Verification items for the finished model (mm, model axes). Face numbers are marked on the shaded views. A direction names the side the tool comes from. Give positions to 0.01 mm unless a question says otherwise; leave off trailing zeros. Write each loop counter-clockwise with the first axis right and the second up, starting at its lowest first coordinate (ties: lowest second). Pieces come first, ordered by that corner, then holes. Notation, with made-up numbers: (-5.5, 29.25) - (10.5, 29.25) arc R4 ccw to (10.5, 36.25) - close; hole circle Ø2 at (23, 31). An arc over 180 degrees is marked (long way). Put each result on its own line as item: value.
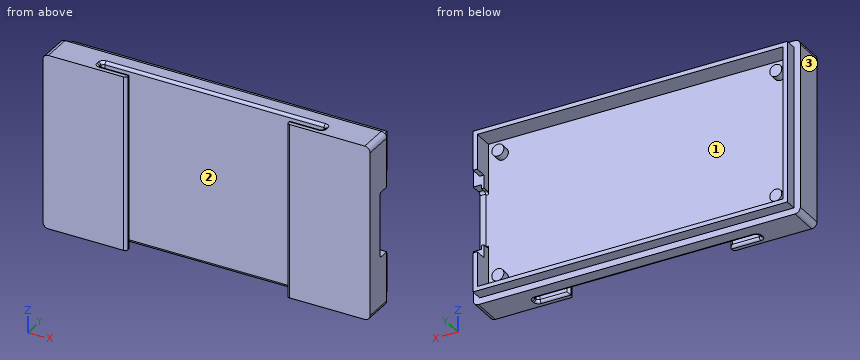
from build123d import *

# Parameters (mm, degrees)
SKETCH2_W               = 61.2
SKETCH2_H               = 32.7
BOSS_EXTRUDE1_DEPTH     = 1.5
BOSS_EXTRUDE2_START     = 1.5
SKETCH2_3_R             = 1.125
BOSS_EXTRUDE2_DEPTH     = 1.5
SKETCH2_4_W             = 61.2
SKETCH2_4_H             = 32.7
BOSS_EXTRUDE3_DEPTH     = 2.5
FILLET1_R               = 1
CUT_EXTRUDE1_DEPTH      = 35.823591142
CUT_EXTRUDE1_DEPTH_BACK = 35.823591142
SKETCH3_W               = 42
SKETCH3_H               = 1.4
SKETCH3_W_2             = 20
SKETCH3_H_2             = 1.25
CUT_EXTRUDE3_DEPTH      = 35.823591142
CUT_EXTRUDE3_DEPTH_BACK = 35.823591142
SKETCH3_4_W             = 5
SKETCH3_4_H             = 1.25
SKETCH3_4_W_2           = 20
FILLET2_R               = 0.5
CUT_EXTRUDE2_START      = 0.75
SKETCH2_5_W             = 1.5
SKETCH2_5_H             = 0.75
SKETCH2_5_H_2           = 10.7
CUT_EXTRUDE2_DEPTH      = 2.25
FILLET3_R               = 0.5
BOSS_EXTRUDE4_DEPTH     = 2.2


with BuildPart() as part:
    # Sketch2 → Boss-Extrude1 (new body)
    with BuildSketch(Plane(origin=(0, 0, 0), x_dir=(1, 0, 0), z_dir=(0, 1, 0))):
        Rectangle(SKETCH2_W, SKETCH2_H)
    extrude(amount=BOSS_EXTRUDE1_DEPTH)

    # Sketch2<3> → Boss-Extrude2 (add)
    with BuildSketch(Plane(origin=(0, 0, 0), x_dir=(1, 0, 0), z_dir=(0, 1, 0)).offset(BOSS_EXTRUDE2_START)):
        Polygon((-30.6, 16.35), (-30.6, -16.35), (30.6, -16.35), (30.6, -6.1), (29.1, -6.1), (29.1, -5.35), (28.6, -5.35), (28.6, -14.35), (-28.6, -14.35), (-28.6, 14.35), (28.6, 14.35), (28.6, 5.35), (30.6, 5.35), (30.6, 16.35), align=None)
        with Locations(Location((-26, 11.75, 0), (0, 0, 270))):
            Circle(SKETCH2_3_R)
        with Locations(Location((-26, -11.75, 0), (0, 0, 270))):
            Circle(SKETCH2_3_R)
        with Locations(Location((26, -11.75, 0), (0, 0, 270))):
            Circle(SKETCH2_3_R)
        with Locations(Location((26, 11.75, 0), (0, 0, 270))):
            Circle(SKETCH2_3_R)
    extrude(amount=BOSS_EXTRUDE2_DEPTH)

    # Sketch2<4> → Boss-Extrude3 (add)
    with BuildSketch(Plane(origin=(0, 0, 0), x_dir=(1, 0, 0), z_dir=(0, 1, 0))):
        Rectangle(SKETCH2_4_W, SKETCH2_4_H)
    extrude(amount=-BOSS_EXTRUDE3_DEPTH)

    # Fillet1
    fillet1_edges = [part.edges().sort_by_distance(p)[0] for p in [
        (-30.6, 0.25, -16.35),
        (30.6, 0.25, -16.35),
        (30.6, 0.25, 16.35),
        (-30.6, 0.25, 16.35),
    ]]
    fillet(fillet1_edges, radius=FILLET1_R)

    # Sketch3 → Cut-Extrude1 (cut, two sides: drawn at the far end of the back side and taken through both)
    with BuildSketch(Plane.XY.offset(-CUT_EXTRUDE1_DEPTH_BACK)):
        with Locations((0, -0.55)):
            Rectangle(SKETCH3_W, SKETCH3_H)
        with Locations((0, -1.875)):
            Rectangle(SKETCH3_W_2, SKETCH3_H_2)
    extrude(amount=CUT_EXTRUDE1_DEPTH + CUT_EXTRUDE1_DEPTH_BACK, mode=Mode.SUBTRACT)

    # Sketch3<4> → Cut-Extrude3 (cut, two sides: drawn at the far end of the back side and taken through both)
    with BuildSketch(Plane.XY.offset(-CUT_EXTRUDE3_DEPTH_BACK)):
        with Locations((12.5, -1.875)):
            Rectangle(SKETCH3_4_W, SKETCH3_4_H)
        with Locations((0, -1.875)):
            Rectangle(SKETCH3_4_W_2, SKETCH3_4_H)
        with Locations((-12.5, -1.875)):
            Rectangle(SKETCH3_4_W, SKETCH3_4_H)
    extrude(amount=CUT_EXTRUDE3_DEPTH + CUT_EXTRUDE3_DEPTH_BACK, mode=Mode.SUBTRACT)

    # Fillet2
    fillet2_edges = [part.edges().sort_by_distance(p)[0] for p in [
        (-18, -1.25, -16.35),
        (-21, -1.25, 0),
        (-21, -0.55, 16.35),
        (-21, 0.15, 0),
        (0, 0.15, 16.35),
        (21, 0.15, 0),
        (21, -0.55, -16.35),
        (21, -1.25, 0),
        (-21, -0.55, -16.35),
        (0, 0.15, -16.35),
        (-18, -1.25, 16.35),
        (21, -0.55, 16.35),
        (18, -1.25, -16.35),
        (18, -1.25, 16.35),
        (-15, -1.25, 0),
        (15, -2.5, 0),
        (-15, -2.5, 0),
        (15, -1.25, 0),
    ]]
    fillet(fillet2_edges, radius=FILLET2_R)

    # Sketch2<5> → Cut-Extrude2 (cut)
    with BuildSketch(Plane(origin=(0, 0, 0), x_dir=(1, 0, 0), z_dir=(0, 1, 0)).offset(CUT_EXTRUDE2_START)):
        with Locations((29.85, 5.725)):
            Rectangle(SKETCH2_5_W, SKETCH2_5_H)
        with Locations((29.85, 0)):
            Rectangle(SKETCH2_5_W, SKETCH2_5_H_2)
        with Locations((29.85, -5.725)):
            Rectangle(SKETCH2_5_W, SKETCH2_5_H)
    extrude(amount=CUT_EXTRUDE2_DEPTH, mode=Mode.SUBTRACT)

    # Fillet3
    fillet3_edges = [part.edges().sort_by_distance(p)[0] for p in [
        (29.85, 0.75, 6.1),
        (29.85, 0.75, -6.1),
        (28.85, 1.5, -5.35),
        (28.85, 1.5, 5.35),
    ]]
    fillet(fillet3_edges, radius=FILLET3_R)

    # Sketch4 → Boss-Extrude4 (add)
    with BuildSketch(Plane(origin=(0, 3, 0), x_dir=(1, 0, 0), z_dir=(0, 1, 0))):
        Polygon((29.4, 15.15), (-29.4, 15.15), (-29.4, -15.15), (29.4, -15.15), (29.4, -7.8), (28.6, -7.8), (28.6, -14.35), (-28.6, -14.35), (-28.6, 14.35), (28.6, 14.35), (28.6, 7.8), (29.4, 7.8), align=None)
    extrude(amount=BOSS_EXTRUDE4_DEPTH)


solid = part.part
Q1. Set-up check for the marked faces 1, 2 and 3: record each of +Z, -Z, +X, -X, +Y, -Y from which the full face is reachable in a straight line by a thin tool's end or side.
Answers follow:
face 1: +Y
face 2: +Z, -Z
face 3: +Z, -Z, -X, +Y, -Y
Q2. Section check A-A, the plane x = -18. Record the cut outline in (y, z), plus the area to 3 significant figures.
Answers follow:
outline: (-2.5, -16.35) - (-1.75, -16.35) arc R0.5 ccw to (-1.25, -15.85) - (-1.25, 15.85) arc R0.5 ccw to (-1.75, 16.35) - (-2.5, 16.35) - close; (0.15, -15.85) arc R0.5 ccw to (0.65, -16.35) - (3, -16.35) - (3, -15.15) - (5.2, -15.15) - (5.2, -14.35) - (1.5, -14.35) - (1.5, 14.35) - (5.2, 14.35) - (5.2, 15.15) - (3, 15.15) - (3, 16.35) - (0.65, 16.35) arc R0.5 ccw to (0.15, 15.85) - close
area: 94.3 mm2
Q3. Section check C-C, the plane x = -3. Record the cut outline in (y, z), plus the area to 3 significant figures.
Answers follow:
outline: (0.15, -15.85) arc R0.5 ccw to (0.65, -16.35) - (3, -16.35) - (3, -15.15) - (5.2, -15.15) - (5.2, -14.35) - (1.5, -14.35) - (1.5, 14.35) - (5.2, 14.35) - (5.2, 15.15) - (3, 15.15) - (3, 16.35) - (0.65, 16.35) arc R0.5 ccw to (0.15, 15.85) - close
area: 53.6 mm2
Q4. Go/stop test with flat-tipped pins: pin 1 Ø1.5 at (x, z) = (18, -4) entering from +Y; pin 2 Ø1.1 at (x, y) = (-6, 3.5) entering from +Z; pin 3 Ø1.5 at (y, z) = (3, -4) entering from +X; pin 4 Ø1.1 at (x, z) = (-26, -11.5) entering from +Y. Record where each tip stops, or that it passes through.
Answers follow:
pin 1: stops at y = 1.5
pin 2: stops at z = 16.35
pin 3: stops at x = -28.6
pin 4: stops at y = 3
Q5. Scan lines: line 1 along X through (y, z) = (2, 6.5); line 2 along Y through (x, z) = (-18.5, -5); line 3 along Z through (x, y) = (-21.5, 4). Record each from-to range of solid material in increasing order.
Answers follow:
line 1: x = -30.6 to -28.6, 28.6 to 30.6
line 2: y = -2.5 to -1.25, 0.15 to 1.5
line 3: z = -15.15 to -14.35, 14.35 to 15.15
Q6. Section check D-D, the plane x = 26. Record the cut outline in (y, z) (3 decimals), plus the area to 3 significant figures.
Answers follow:
outline: (-2.5, -16.35) - (3, -16.35) - (3, -15.15) - (5.2, -15.15) - (5.2, -14.35) - (1.5, -14.35) - (1.5, -12.875) - (3, -12.875) - (3, -10.625) - (1.5, -10.625) - (1.5, 10.625) - (3, 10.625) - (3, 12.875) - (1.5, 12.875) - (1.5, 14.35) - (5.2, 14.35) - (5.2, 15.15) - (3, 15.15) - (3, 16.35) - (-2.5, 16.35) - close
area: 147 mm2
Q7. Section check B-B, the plane y = 3.75. Record the cut outline in (x, z), plus the area to 3 significant figures.
Answers follow:
outline: (-29.4, -15.15) - (29.4, -15.15) - (29.4, -7.8) - (28.6, -7.8) - (28.6, -14.35) - (-28.6, -14.35) - (-28.6, 14.35) - (28.6, 14.35) - (28.6, 7.8) - (29.4, 7.8) - (29.4, 15.15) - (-29.4, 15.15) - close
area: 128 mm2
